For this review, take the finished solid that the model builds, in its own axes (mm). Round coordinates to 2 decimals unless told otherwise and drop trailing zeros. Write each loop counter-clockwise with the first axis right and the second up, starting at its lowest first coordinate (ties: lowest second). Pieces come first, ordered by that corner, then holes. Notation, with made-up numbers: (-7, 50) - (12, 50) arc R25 cw to (12, 70) - close; hole circle Ø3 at (-27.5, -32.75). An arc over 180 degrees is marked (long way). One line per item, written item: value. Start each with the question number.
Q1. Add section B-B on z = 5. Give the number of separate pieces and of enclosed holes in the cut face, and give its area (3 significant figures).
Q2. Clearance check with a flat-ended pin moving along its axis: pin 1 Ø5 at (x, y) = (163.53, -67.73) entering from -Z. State where the tip first meets the part, or that it passes through.
Q3. Add section C-C on x = -15. Write out the cut boundary in (y, z) (3 decimals).
Q4. For probe 1 along Y at (x, z) = (-69.5, 1) (3 decimals); probe 2 along Y at (x, z) = (68.5, 1.25) (3 decimals); probe 3 along Y at (x, z) = (-162.5, 5.5) (3 decimals), list the stretches that pass through material, from the lowest coordinate up.
Q5. Add section A-A on y = -54. Write out the cut boundary in (x, z) (3 decimals).
Q6. Mouldability with a two-part tool opening along Y and no side actions: class faces 1 (the face through (-3, -199.995, 10)), 2 (the face through (-33.601, -151.314, 10.14)), 3 (the face through (-3, 199.995, 10)) as +Y half, -Y half, draft (parallel to the pull), parting line (faces both ways), or undercut.
```python
from build123d import *

# Parameters (mm, degrees)
SKETCH_W           = 399.99
SKETCH_H           = 399.99
PAD_DEPTH          = 20
SKETCH001_R        = 155
POCKET_DEPTH       = 20.001
SKETCH002_R        = 2
POCKET001_DEPTH    = 1152.050469
POLARPATTERN_COUNT = 16


with BuildPart() as part:
    # Sketch → Pad (new body)
    with BuildSketch(Plane.XY):
        Rectangle(SKETCH_W, SKETCH_H)
    extrude(amount=PAD_DEPTH)

    # Sketch001 (on Face6 of Pad) → Pocket (cut, through all)
    with BuildSketch(Plane.XY.offset(20)):
        Circle(SKETCH001_R)
    extrude(amount=-POCKET_DEPTH, mode=Mode.SUBTRACT)

    # Sketch002 (on Face5 of Pocket) → Pocket001 (cut, through all)
    with BuildSketch(Plane.XY.offset(20)):
        with Locations((0, 177)):
            Circle(SKETCH002_R)
    pocket001 = extrude(amount=-POCKET001_DEPTH, mode=Mode.SUBTRACT)

    # PolarPattern: Pocket001 ×16 about axis
    polarpattern_axis = Axis((0, 0, 20), (0, 0, 1))
    for i in range(1, POLARPATTERN_COUNT):
        add(pocket001.rotate(polarpattern_axis, i * 360 / POLARPATTERN_COUNT), mode=Mode.SUBTRACT)


solid = part.part
```
Result set:
1. separate pieces: 1
1. enclosed holes: 17
1. area: 84,300 mm^2
2. pin 1: stops at z = 0
3. outline: (-199.995, 0) - (-154.272, 0) - (-154.272, 20) - (-199.995, 20) - close; (154.272, 0) - (199.995, 0) - (199.995, 20) - (154.272, 20) - close
4. probe 1: y = -199.995 to -164.467, -162.586 to -138.545, 138.545 to 162.586, 164.467 to 199.995
4. probe 2: y = -199.995 to -165.375, -161.679 to -139.042, 139.042 to 161.679, 165.375 to 199.995
4. probe 3: y = -199.995 to -69.451, -66.019 to 66.019, 69.451 to 199.995
5. outline: (-199.995, 0) - (-145.289, 0) - (-145.289, 20) - (-199.995, 20) - close; (145.289, 0) - (199.995, 0) - (199.995, 20) - (145.289, 20) - close
6. face 1: -Y half
6. face 2: undercut
6. face 3: +Y half
